Can you work these out from the model? Positions are in its coordinate system, mm. A direction names the side the tool comes from. Give positions to 0.01 mm unless a question says otherwise; leave off trailing zeros. Write each loop counter-clockwise with the first axis right and the second up, starting at its lowest first coordinate (ties: lowest second). Pieces come first, ordered by that corner, then holes. Notation, with made-up numbers: M 77,53.25 L 135,53.25 A24 ccw 135,68.25 Z; hole C 79,-8.75 d5. An arc over 180 degrees is marked long. Use CSV: the item, a comma, the result in double quotes. Start each with the question number.
from build123d import *

# Parameters (mm, degrees)
F1_DEPTH = 30.4
F2_DEPTH = 2
F3_W     = 6.9
F3_H     = 6.9
F4_DEPTH = 50
F5_R     = 1


# Not quite as in the source:
# - a feature of the source that left no trace in its solid (it failed there, or was rolled back) is left out
# - a feature names something its author has since deleted; it is built from what else it names


with BuildPart() as f1:
    # F0 (on Top) → F1 (new body)
    with BuildSketch(Plane.XY):
        with BuildLine():
            ThreePointArc((0, -18), (-18, 0), (0, 18))
            Line((0, 18), (-27.8, 18))
            Line((-27.8, 18), (-27.8, -18))
            Line((-27.8, -18), (0, -18))
        make_face()
        with BuildLine():
            ThreePointArc((0, -11.2), (-11.2, 0), (0, 11.2))
            Line((0, 11.2), (0, 18))
            ThreePointArc((0, 18), (-18, 0), (0, -18))
            Line((0, -18), (0, -11.2))
        make_face()
        with BuildLine():
            ThreePointArc((0, 11.2), (7.9195959493, 7.9195959493), (11.2, 0))
            ThreePointArc((11.2, 0), (7.9195959493, -7.9195959493), (0, -11.2))
            Line((0, -11.2), (0, -18))
            ThreePointArc((0, -18), (12.7279220614, -12.7279220614), (18, 0))
            ThreePointArc((18, 0), (12.7279220614, 12.7279220614), (0, 18))
            Line((0, 18), (0, 11.2))
        make_face()
    extrude(amount=F1_DEPTH)

    # F0 (on Top) → F2 (join)
    with BuildSketch(Plane.XY):
        with BuildLine():
            ThreePointArc((0, -11.2), (7.9195959493, -7.9195959493), (11.2, 0))
            ThreePointArc((11.2, 0), (7.9195959493, 7.9195959493), (0, 11.2))
            Line((0, 11.2), (0, 5))
            ThreePointArc((0, 5), (3.5355339059, 3.5355339059), (5, 0))
            ThreePointArc((5, 0), (3.5355339059, -3.5355339059), (0, -5))
            Line((0, -5), (0, -11.2))
        make_face()
        with BuildLine():
            Line((0, 5), (0, 11.2))
            ThreePointArc((0, 11.2), (-11.2, 0), (0, -11.2))
            Line((0, -11.2), (0, -5))
            ThreePointArc((0, -5), (-5, 0), (0, 5))
        make_face()
    extrude(amount=F2_DEPTH)

    # F3 (on face) → F4 (cut)
    with BuildSketch(Plane.XZ.offset(18)):
        with Locations((-22.45, 25.05)):
            Rectangle(F3_W, F3_H)
        with Locations((-22.45, 5.35)):
            Rectangle(F3_W, F3_H)
    extrude(amount=-F4_DEPTH, mode=Mode.SUBTRACT)

    # F5
    f5_edges = [f1.edges().sort_by_distance(p)[0] for p in [
        (-27.8, 18, 15.2),
        (-27.8, -18, 15.2),
    ]]
    fillet(f5_edges, radius=F5_R)


solid = f1.part
(1) I want a section at A-A (z = 5.5). Write out the boundary of the cut face in (x, y).
(2) I want a section at D-D (y = -9). Write out the boundary of the cut face in (x, z).
(3) I want a section at B-B (x = -23). Write out the boundary of the cut face in (y, z), and give its area (3 significant figures).
(4) Please list where these lines run through material, in increasing order: L1, parallel to Z at x = -20.5, y = 8.5; L2, parallel to X at y = -2.5, z = 2.5; L3, parallel to Z at x = -6, y = -8.5. Write a range as [from, to].
(5) Thinking about a two-plate mould opening in Z: for faces 4 (the face through (-5.2, 0.3, 0)), 5 (the face through (-27.499, 17.715, 15.413)), 6 (the face through (-22, 0, 1.9)), which applies, released by +Z, released by -Z, zero draft, split by the parting line, or undercut?
(6) Which directions (+Z, -Z, +X, -X, +Y, -Y) give clear straight access to the entire face, cutting with the end or side of a thin tool? Please do faces 1 (the face through (-22, 0, 8.8)), 2 (the face through (5, -2, 2)), 3 (the face through (-27.515, -17.699, 15.413)).
(7) Will these pins go through, and if not, where does the flat tip stop? pin 1 Ø8 at (y, z) = (-3, 15) entering from +X; pin 2 Ø2 at (y, z) = (8.5, 17.5) entering from +X; pin 3 Ø5.5 at (y, z) = (6, 5) entering from +X.
(8) I want a section at C-C (z = 18). Write out the boundary of the cut face in (x, y), and give its area (3 significant figures).
Geometry results:
1,outline,"M -27.8,-17 A1 ccw -26.8,-18 L -25.9,-18 L -25.9,18 L -26.8,18 A1 ccw -27.8,17 Z; M -19,-18 L 0,-18 A18 ccw 0,18 L -19,18 Z; hole C 0,0 d22.4"
2,outline,"M -27.8,0 L 15.59,0 L 15.59,30.4 L 6.67,30.4 L 6.67,2 L -6.67,2 L -6.67,30.4 L -27.8,30.4 Z; hole M -25.9,1.9 L -19,1.9 L -19,8.8 L -25.9,8.8 Z; hole M -25.9,21.6 L -19,21.6 L -19,28.5 L -25.9,28.5 Z"
3,outline,"M -18,0 L 18,0 L 18,1.9 L -18,1.9 Z; M -18,8.8 L 18,8.8 L 18,21.6 L -18,21.6 Z; M -18,28.5 L 18,28.5 L 18,30.4 L -18,30.4 Z"
3,area,"598 mm2"
4,L1,"z = [0, 1.9], [8.8, 21.6], [28.5, 30.4]"
4,L2,"x = [-27.8, -25.9], [-19, -10.92], [10.92, 17.83]"
4,L3,"z = [0, 2]"
5,face 4,"released by -Z"
5,face 5,"zero draft"
5,face 6,"undercut"
6,face 1,"+Y, -Y"
6,face 2,"+Z"
6,face 3,"+Z, -Z, -X, -Y"
7,pin 1,"stops at x = 18"
7,pin 2,"stops at x = 16.36"
7,pin 3,"stops at x = 17.7"
8,outline,"M -27.8,-17 A1 ccw -26.8,-18 L 0,-18 A18 ccw 0,18 L -26.8,18 A1 ccw -27.8,17 Z; hole C 0,0 d22.4"
8,area,"1,120 mm2"
